```python
from build123d import *

# Parameters (mm, degrees)
SKETCH1_W           = 200
SKETCH1_H           = 100
SKETCH1_R           = 2.5
BOSS_EXTRUDE1_DEPTH = 5
SKETCH2_R           = 2.5
CUT_EXTRUDE1_DEPTH  = 5
SKETCH4_W           = 150
SKETCH4_H           = 40
CUT_EXTRUDE3_DEPTH  = 30


with BuildPart() as part:
    # Sketch1 → Boss-Extrude1 (new body)
    with BuildSketch(Plane.XY):
        Rectangle(SKETCH1_W, SKETCH1_H)
        with Locations((-92.5, 42.5)):
            Circle(SKETCH1_R, mode=Mode.SUBTRACT)
        with Locations((-57.5, 42.5)):
            Circle(SKETCH1_R, mode=Mode.SUBTRACT)
        with Locations((57.5, -42.5)):
            Circle(SKETCH1_R, mode=Mode.SUBTRACT)
        with Locations((92.5, -42.5)):
            Circle(SKETCH1_R, mode=Mode.SUBTRACT)
        with Locations((57.5, 42.5)):
            Circle(SKETCH1_R, mode=Mode.SUBTRACT)
        with Locations((92.5, 42.5)):
            Circle(SKETCH1_R, mode=Mode.SUBTRACT)
        with Locations((-87.5, -37.5)):
            Circle(SKETCH1_R, mode=Mode.SUBTRACT)
        with Locations((-52.5, -37.5)):
            Circle(SKETCH1_R, mode=Mode.SUBTRACT)
    extrude(amount=BOSS_EXTRUDE1_DEPTH)

    # Sketch2 → Cut-Extrude1 (cut)
    with BuildSketch(Plane.XY.offset(5)):
        with Locations((-87.5, -2.5)):
            Circle(SKETCH2_R)
        with Locations((-52.5, -2.5)):
            Circle(SKETCH2_R)
        with Locations((-87.5, -37.5)):
            Circle(SKETCH2_R)
        with Locations((-52.5, -37.5)):
            Circle(SKETCH2_R)
    extrude(amount=-CUT_EXTRUDE1_DEPTH, mode=Mode.SUBTRACT)

    # Sketch4 → Cut-Extrude3 (cut)
    with BuildSketch(Plane.XY.offset(5)):
        with Locations((-25, 30)):
            Rectangle(SKETCH4_W, SKETCH4_H)
    extrude(amount=-CUT_EXTRUDE3_DEPTH, mode=Mode.SUBTRACT)


solid = part.part
```
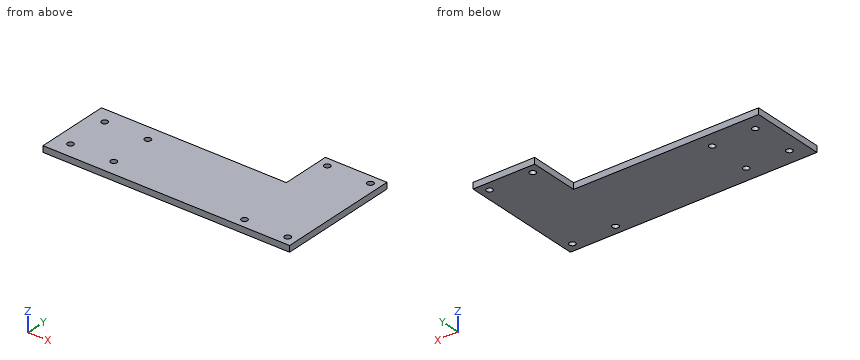
The listing builds one solid part. Answer for the finished solid, in the listing's coordinates (mm). Coordinates: 2 decimals unless noted, no trailing zeros. Write each loop counter-clockwise with the first axis right and the second up, starting at its lowest first coordinate (ties: lowest second). Pieces come first, ordered by that corner, then holes. Notation, with made-up numbers: M 86,-30 L 95,-30 A34 ccw 95,4 Z; hole C -9,73.25 d5. An arc over 180 degrees is marked long. Use a Markdown table: item, result. Add a question column.
1. Section C-C (y = 42.5) is taken. Give the vertices of the cut face in (x, z).
2. Section A-A (x = -52.5) is taken. Give the vertices of the cut face in (y, z), plus the area to 3 significant figures.
3. Straight lines are drawn through the part: line 1 along Y through (x, z) = (92.5, 1.55); line 2 along Y through (x, z) = (-87.5, 2.85); line 3 along Y through (x, z) = (45, 1.5). For each, find the intervals that lie inside material, in ascending order. Write a range as [from, to].
4. Section D-D (x = -79.5) is taken. Give the vertices of the cut face in (y, z).
5. Section B-B (z = 1.7) is taken. Count the separate pieces of the cut face and the enclosed holes in it, plus the area to 3 significant figures.
6. Given P1, Ø4.5, axis at x = -52.5, y = -2.5, coming from the +Z side; P2, Ø2, axis at x = 7, z = 1, coming from the +Y side, each flat-ended and moving along its own axis, determine where each tip first touches the part or whether it passes through.
Data:
| question | item | result |
|---|---|---|
| 1 | outline | M 50,0 L 55,0 L 55,5 L 50,5 Z; M 60,0 L 90,0 L 90,5 L 60,5 Z; M 95,0 L 100,0 L 100,5 L 95,5 Z |
| 2 | outline | M -50,0 L -40,0 L -40,5 L -50,5 Z; M -35,0 L -5,0 L -5,5 L -35,5 Z; M 0,0 L 10,0 L 10,5 L 0,5 Z |
| 2 | area | 250 mm2 |
| 3 | line 1 | y = [-50, -45], [-40, 40], [45, 50] |
| 3 | line 2 | y = [-50, -40], [-35, -5], [0, 10] |
| 3 | line 3 | y = [-50, 10] |
| 4 | outline | M -50,0 L 10,0 L 10,5 L -50,5 Z |
| 5 | separate pieces | 1 |
| 5 | enclosed holes | 8 |
| 5 | area | 13,800 mm2 |
| 6 | P1 | passes through |
| 6 | P2 | stops at y = 10 |
